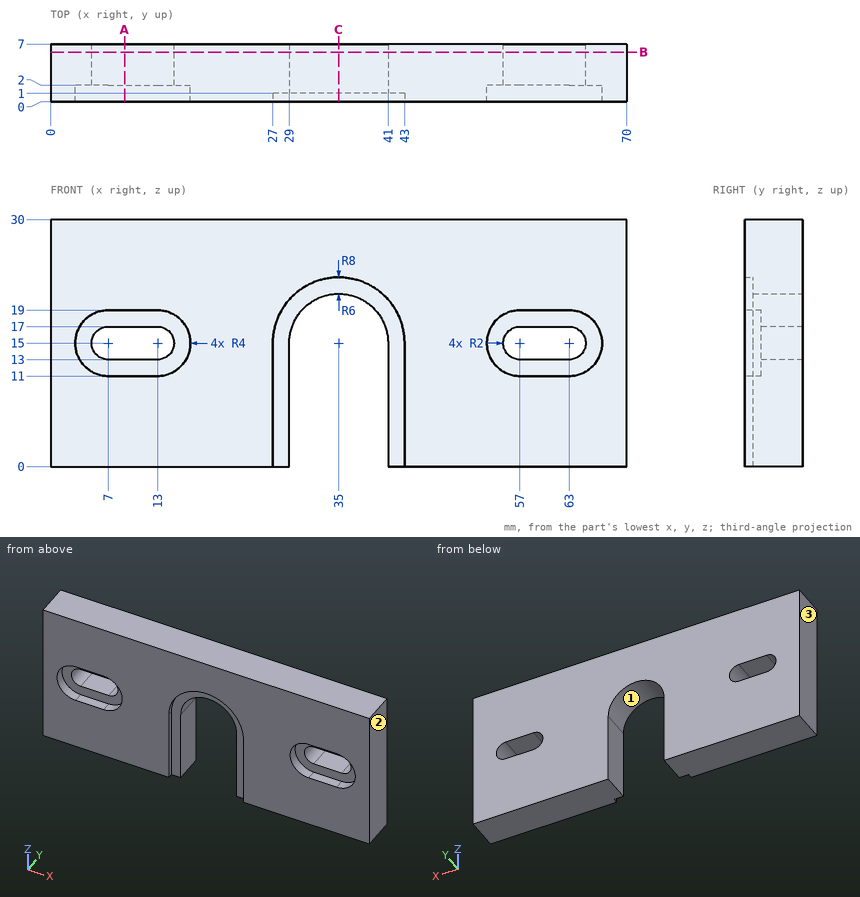
The drawing under review shows one solid part. Ordinate dimensions are in mm from its lowest x, y, z. Round coordinates to 2 decimals unless told otherwise and drop trailing zeros. Write each loop counter-clockwise with the first axis right and the second up, starting at its lowest first coordinate (ties: lowest second). Pieces come first, ordered by that corner, then holes. Notation, with made-up numbers: (25, -6) -> (33, -6) arc R23 cw to (33, 29) -> close; hole circle Ø7 at (37.5, 18.25). An arc over 180 degrees is marked (long way). One line per question, with ' | ' between items. Start each with the question number.
(1) Add section A-A, the plane x = 9. Write out the cut boundary in (y, z), plus the area to 3 significant figures.
(2) Add section B-B, the plane y = 6. Write out the cut boundary in (x, z), plus the area to 3 significant figures.
(3) Add section C-C, the plane x = 35. Write out the cut boundary in (y, z), plus the area to 3 significant figures.
(4) Mouldability with a two-part tool opening along X and no side actions: class the marked faces 1, 2 and 3 as released by +X, released by -X, zero draft, split by the parting line, or undercut.
(5) For line 1 along X through (y, z) = (4, 5.5); line 2 along Z through (x, y) = (7, 5.5); line 3 along X through (y, z) = (3.5, 15.25), list the stretches that pass through material, from the lowest coordinate up. Write a range as from..to.
Answer list:
1) outline: (0, 0) -> (7, 0) -> (7, 13) -> (2, 13) -> (2, 11) -> (0, 11) -> close; (0, 19) -> (2, 19) -> (2, 17) -> (7, 17) -> (7, 30) -> (0, 30) -> close | area: 174 mm²
2) outline: (0, 0) -> (29, 0) -> (29, 15) arc R6 cw to (41, 15) -> (41, 0) -> (70, 0) -> (70, 30) -> (0, 30) -> close; hole (7, 13) -> (13, 13) arc R2 ccw to (13, 17) -> (7, 17) arc R2 ccw to start; hole (57, 13) -> (63, 13) arc R2 ccw to (63, 17) -> (57, 17) arc R2 ccw to start | area: 1,790 mm²
3) outline: (0, 23) -> (1, 23) -> (1, 21) -> (7, 21) -> (7, 30) -> (0, 30) -> close | area: 61.0 mm²
4) face 1: undercut | face 2: released by +X | face 3: released by -X
5) line 1: 0..29, 41..70 | line 2: 0..13, 17..30 | line 3: 0..5.02, 14.98..29.01, 40.99..55.02, 64.98..70
